from build123d import *

# Parameters (mm, degrees)
SKETCH1_W           = 101.6
SKETCH1_H           = 127
BOSS_EXTRUDE1_DEPTH = 5
SKETCH4_W           = 102.6
SKETCH4_H           = 128
BOSS_EXTRUDE3_DEPTH = 5
SKETCH5_W           = 112.6
SKETCH5_H           = 138
SKETCH5_W_2         = 102.6
SKETCH5_H_2         = 128
BOSS_EXTRUDE4_DEPTH = 50


with BuildPart() as part:
    # Sketch1 → Boss-Extrude1 (new body)
    with BuildSketch(Plane(origin=(0, 0, 0), x_dir=(1, 0, 0), z_dir=(0, 1, 0))):
        with Locations((9.420607765, 19.952255333)):
            Rectangle(SKETCH1_W, SKETCH1_H)
    extrude(amount=BOSS_EXTRUDE1_DEPTH)

    # Sketch4 → Boss-Extrude3 (add)
    with BuildSketch(Plane(origin=(0, 5, 0), x_dir=(1, 0, 0), z_dir=(0, 1, 0))):
        with Locations((9.420607765, 19.952255333)):
            Rectangle(SKETCH4_W, SKETCH4_H)
    extrude(amount=-BOSS_EXTRUDE3_DEPTH)

    # Sketch5 → Boss-Extrude4 (add)
    with BuildSketch(Plane.XZ):
        with Locations((9.420607765, -19.952255333)):
            Rectangle(SKETCH5_W, SKETCH5_H)
        with Locations((9.420607765, -19.952255333)):
            Rectangle(SKETCH5_W_2, SKETCH5_H_2, mode=Mode.SUBTRACT)
    extrude(amount=-BOSS_EXTRUDE4_DEPTH)


solid = part.part
The listing builds one solid part. Answer for the finished solid, in the listing's coordinates (mm). A direction names the side the tool comes from. Give positions to 0.01 mm unless a question says otherwise; leave off trailing zeros. Write each loop counter-clockwise with the first axis right and the second up, starting at its lowest first coordinate (ties: lowest second). Pieces come first, ordered by that corner, then holes. Notation, with made-up numbers: (79.25, 62.25) - (112.25, 62.25) arc R31 cw to (112.25, 92.25) - close; hole circle Ø3 at (3, 34). An arc over 180 degrees is marked (long way). Use a Markdown table: item, result.
1. Find the intervals of material crossed by probe 1 along X at (y, z) = (42.5, 7.5); probe 2 along Z at (x, y) = (-23.5, 19); probe 3 along Y at (x, z) = (12, -64), in increasing order. Write a range as from..to.
Values follow:
| item | result |
|---|---|
| probe 1 | x = -46.88..-41.88, 60.72..65.72 |
| probe 2 | z = -88.95..-83.95, 44.05..49.05 |
| probe 3 | y = 0..5 |
2. Section A-A on z = 33.5 is taken. Write down the section's boundary in (x, y), plus the area to 3 significant figures.
Values follow:
| item | result |
|---|---|
| outline | (-46.88, 0) - (65.72, 0) - (65.72, 50) - (60.72, 50) - (60.72, 5) - (-41.88, 5) - (-41.88, 50) - (-46.88, 50) - close |
| area | 1,010 mm² |
3. Section B-B on y = 45 is taken. Write down the section's boundary in (x, z), plus the area to 3 significant figures.
Values follow:
| item | result |
|---|---|
| outline | (-46.88, -88.95) - (65.72, -88.95) - (65.72, 49.05) - (-46.88, 49.05) - close; hole (-41.88, -83.95) - (60.72, -83.95) - (60.72, 44.05) - (-41.88, 44.05) - close |
| area | 2,410 mm² |
4. Section C-C on x = -28.5 is taken. Write down the section's boundary in (y, z), plus the area to 3 significant figures.
Values follow:
| item | result |
|---|---|
| outline | (0, -88.95) - (50, -88.95) - (50, -83.95) - (5, -83.95) - (5, 44.05) - (50, 44.05) - (50, 49.05) - (0, 49.05) - close |
| area | 1,140 mm² |
5. A tool of negligible diameter and unlimited length cuts with its end or side. For faces 5 (the flat face through (-45, 50, -20)), 6 (the flat face through (9, 5, -21)), from which of +Z, -Z, +X, -X, +Y, -Y can it reach the whole face along a straight path? Write none if from no direction.
Values follow:
| item | result |
|---|---|
| face 5 | +Z, -Z, +X, -X, +Y |
| face 6 | +Y |
6. For a pull along Z with two mould halves and no side action, classify faces 1 (the flat face through (-46.879, 25, -21)), 2 (the flat face through (9, 27, 44.048)), 3 (the flat face through (9, 25, -88.952)), 4 (the flat face through (60.721, 27, -21)) as released by +Z, released by -Z, zero draft, split by the parting line, or undercut.
Values follow:
| item | result |
|---|---|
| face 1 | zero draft |
| face 2 | undercut |
| face 3 | released by -Z |
| face 4 | undercut |
7. This flat-tipped pin is pushed along its axis until it touches: P1, Ø2, axis at x = -27.5, z = 7.5, coming from the +Y side. Where does it stop, or does it pass through?
Values follow:
| item | result |
|---|---|
| P1 | stops at y = 5 |
